Source: CAD feature listing. Evaluate the final solid. Frame: model axes, mm. A direction names the side the tool comes from. Coordinates: 2 decimals unless noted, no trailing zeros. Loops run counter-clockwise (first coordinate to the right, second up) from the corner with the lowest first, then second, coordinate; pieces in that order, holes last.
from build123d import *

# Parameters (mm, degrees)
SKETCH1_W           = 9.525
SKETCH1_H           = 7.9248
BOSS_EXTRUDE1_DEPTH = 1.016
SKETCH2_W           = 1.016
SKETCH2_H           = 7.9248
BOSS_EXTRUDE2_DEPTH = 0.635
SKETCH3_W           = 1.016
SKETCH3_H           = 1.8542
SKETCH3_H_2         = 1.016
BOSS_EXTRUDE3_DEPTH = 4.7498
CHAMFER1_SIZE       = 0.254
SKETCH4_R           = 0.381
BOSS_EXTRUDE4_DEPTH = 5.3848
FILLET1_R           = 0.254
BOSS_EXTRUDE5_START = 8.001
SKETCH5_R           = 1.5875
SKETCH5_R_2         = 1.27
SKETCH5_R_3         = 0.381
BOSS_EXTRUDE5_DEPTH = 8.001
SKETCH7_R           = 0.381
CUT_EXTRUDE1_DEPTH  = 1.524
SKETCH8_R           = 0.381
BOSS_EXTRUDE6_DEPTH = 0.762
BOSS_EXTRUDE6_TAPER = 15
FILLET2_R           = 0.127
FILLET3_R           = 0.127


with BuildPart() as part:
    # Sketch1 → Boss-Extrude1 (new body)
    with BuildSketch(Plane(origin=(0, 0, 0), x_dir=(1, 0, 0), z_dir=(0, 1, 0))):
        Rectangle(SKETCH1_W, SKETCH1_H)
    extrude(amount=BOSS_EXTRUDE1_DEPTH)

    # Sketch2 → Boss-Extrude2 (add)
    with BuildSketch(Plane(origin=(0, 1.016, 0), x_dir=(1, 0, 0), z_dir=(0, 1, 0))):
        with Locations((-4.2545, 0)):
            Rectangle(SKETCH2_W, SKETCH2_H)
        with Locations((4.2545, 0)):
            Rectangle(SKETCH2_W, SKETCH2_H)
    extrude(amount=BOSS_EXTRUDE2_DEPTH)

    # Sketch3 → Boss-Extrude3 (add)
    with BuildSketch(Plane(origin=(0, 1.651, 0), x_dir=(1, 0, 0), z_dir=(0, 1, 0))):
        with Locations((-4.2545, -3.0353)):
            Rectangle(SKETCH3_W, SKETCH3_H)
        with Locations((-4.2545, 0.127)):
            Rectangle(SKETCH3_W, SKETCH3_H_2)
        with Locations((4.2545, 0.127)):
            Rectangle(SKETCH3_W, SKETCH3_H_2)
        with Locations((4.2545, -3.0353)):
            Rectangle(SKETCH3_W, SKETCH3_H)
    extrude(amount=BOSS_EXTRUDE3_DEPTH)

    # Chamfer1
    chamfer1_edges = [part.edges().sort_by_distance(p)[0] for p in [
        (-4.2545, 6.4008, 2.1082),
        (-4.2545, 6.4008, 0.381),
        (4.2545, 6.4008, 0.381),
        (4.2545, 6.4008, 2.1082),
    ]]
    chamfer(chamfer1_edges, length=CHAMFER1_SIZE)

    # Sketch4 → Boss-Extrude4 (add)
    with BuildSketch(Plane(origin=(0, 1.016, 0), x_dir=(1, 0, 0), z_dir=(0, 1, 0))):
        with Locations(Location((0, 0, 0), (0, 0, 90))):
            Circle(SKETCH4_R)
    extrude(amount=BOSS_EXTRUDE4_DEPTH)

    # Fillet1
    fillet1_edges = [part.edges().sort_by_distance(p)[0] for p in [
        (0, 6.4008, 0.381),
    ]]
    fillet(fillet1_edges, radius=FILLET1_R)

    # Sketch5 → Boss-Extrude5 (add)
    # profile 1 of 2: a face of its own
    with BuildSketch(Plane.XZ.offset(BOSS_EXTRUDE5_START)):
        with Locations(Location((0, 0, 0), (0, 0, 270))):
            Circle(SKETCH5_R)
        with Locations(Location((0, 0, 0), (0, 0, 270))):
            Circle(SKETCH5_R_2, mode=Mode.SUBTRACT)
    # profile 2 of 2: a face of its own
    with BuildSketch(Plane.XZ.offset(BOSS_EXTRUDE5_START)):
        with Locations(Location((0, 0, 0), (0, 0, 270))):
            Circle(SKETCH5_R_3)
    extrude(amount=-BOSS_EXTRUDE5_DEPTH)

    # Sketch6 → Cut-Revolve1 (revolve, cut)
    with BuildSketch(Plane(origin=(0, 0, 0), x_dir=(0, 0, -1), z_dir=(1, 0, 0))):
        Polygon((1.5875, -4.5085), (1.4605, -4.6355), (1.4605, -4.7625), (1.5875, -4.8895), align=None)
    revolve(axis=Axis((0, -8.001, 0), (0, 1, 0)), mode=Mode.SUBTRACT)

    # Sketch7 → Cut-Extrude1 (cut)
    with BuildSketch(Plane.XZ.offset(8.001)):
        with Locations(Location((0, 0, 0), (0, 0, 270))):
            Circle(SKETCH7_R)
    extrude(amount=-CUT_EXTRUDE1_DEPTH, mode=Mode.SUBTRACT)

    # Sketch8 → Boss-Extrude6 (add)
    with BuildSketch(Plane.XZ.offset(6.477)):
        with Locations(Location((0, 0, 0), (0, 0, 270))):
            Circle(SKETCH8_R)
    extrude(amount=BOSS_EXTRUDE6_DEPTH, taper=BOSS_EXTRUDE6_TAPER)

    # Fillet2
    fillet2_edges = [part.edges().sort_by_distance(p)[0] for p in [
        (0, -7.239, 0.176822715),
    ]]
    fillet(fillet2_edges, radius=FILLET2_R)

    # Fillet3
    fillet3_edges = [part.edges().sort_by_distance(p)[0] for p in [
        (0, -8.001, 1.5875),
    ]]
    fillet(fillet3_edges, radius=FILLET3_R)


solid = part.part
Q1. Section B-B, the plane z = -2. Return the cut outline in (x, y).
Q2. Section C-C, the plane x = -4. Return the cut outline in (y, z) (3 decimals), plus the area to 3 significant figures.
Q3. Section A-A, the plane y = 2.75. Return the cut outline in (x, z) (1 decimal), plus the area to 3 significant figures.
Q4. Contact query for flat-ended pins moving along their axis: pin 1 Ø0.8 at (x, y) = (4, 3) entering from -Z (3 decimals); pin 2 Ø1.1 at (x, z) = (-4, 1) entering from +Y. Output: stop coordinate, or through.
Q5. Section D-D, the plane y = -3.75. Return the cut outline in (x, z) (1 decimal).
Q6. Access query for faces 1 (the flat face through (-3.746, 3, 3)), 2 (the cylindrical face through (-0.966, -6.403, 1.26)), 3 (the flat face through (4, 4, 2.108)), 4 (the flat face through (-4, 6.401, 3)), 5 (the flat face through (4, 4, -0.635)). Directions: +Z, -Z, +X, -X, +Y, -Y. A direction counts if a zero-diameter tool reaches every point of the face in a straight line with its end or side. Return the directions, or none.
Q7. Line query: line 1 along X through (y, z) = (-5.25, 0); line 2 along X through (y, z) = (3.5, 0); line 3 along X through (y, z) = (1.5, -1.5). Output: solid intervals per line, ascending.
Derived:
1. outline: (-4.76, 0) - (4.76, 0) - (4.76, 1.65) - (3.75, 1.65) - (3.75, 1.02) - (-3.75, 1.02) - (-3.75, 1.65) - (-4.76, 1.65) - close
2. outline: (0, -3.962) - (1.651, -3.962) - (1.651, -0.635) - (6.401, -0.635) - (6.401, 0.127) - (6.147, 0.381) - (1.651, 0.381) - (1.651, 2.108) - (6.147, 2.108) - (6.401, 2.362) - (6.401, 3.962) - (0, 3.962) - close
2. area: 26.7 mm2
3. outline: (-4.8, -0.6) - (-3.7, -0.6) - (-3.7, 0.4) - (-4.8, 0.4) - close; (-4.8, 2.1) - (-3.7, 2.1) - (-3.7, 4) - (-4.8, 4) - close; circle Ø0.8 at (0, 0); (3.7, -0.6) - (4.8, -0.6) - (4.8, 0.4) - (3.7, 0.4) - close; (3.7, 2.1) - (4.8, 2.1) - (4.8, 4) - (3.7, 4) - close
3. area: 6.29 mm2
4. pin 1: stops at z = -0.635
4. pin 2: stops at y = 1.65
5. outline: circle Ø3.2 at (0, 0); circle Ø0.8 at (0, 0); hole circle Ø2.5 at (0, 0)
6. face 1: +Z, -Z, +Y
6. face 2: -Y
6. face 3: +X, -X, +Y
6. face 4: +Z, -Z, +X, -X, +Y
6. face 5: -Z, +X, -X, +Y
7. line 1: x = -1.59 to -1.27, -0.38 to 0.38, 1.27 to 1.59
7. line 2: x = -4.76 to -3.75, -0.38 to 0.38, 3.75 to 4.76
7. line 3: x = -4.76 to -3.75, 3.75 to 4.76
